Autodesk Inventor part; units mm, degrees
ref_plane "Work Plane1" through (0, 3.95, 0) normal (0, 1, 0) x (1, 0, 0)
ref_plane "Work Plane2" through (0, 4.1, 0) normal (0, 1, 0) x (1, 0, 0)
ref_plane "YZ Plane" through (0, 0, 0) normal (1, 0, 0) x (0, 1, 0)
sketch "Sketch1" plane through (0, 0, 0) normal (0, 1, 0) x (-1, 0, 0)
  circle A0 centre (0, 0) radius 2.5
  circle A1 centre (0, 0) radius 3.65
  dimension "d0" = 5
  dimension "d1" = 7.3
extrude "Extrusion1" add sketch "Sketch1" along normal blind 5.2
ref_plane "Work Plane1" through (0, 3.95, 0) normal (0, 1, 0) x (1, 0, 0)
sketch "Sketch2" plane through (0, 3.95, 0) normal (0, 1, 0) x (1, 0, 0)
  circle A0 centre (0, 0) radius 2.5
  circle A1 centre (0, 0) radius 1.2
  dimension "d5" = 2.4
extrude "Extrusion2" add sketch "Sketch2" against normal blind 1
ref_plane "Work Plane2" through (0, 4.1, 0) normal (0, 1, 0) x (1, 0, 0)
sketch "Sketch3" plane through (0, 4.1, 0) normal (0, 1, 0) x (1, 0, 0)
  line L0 (5.5656, 0) -> (-5.5656, 0) construction
  circle A0 centre (0, 16.05) radius 2
  line L1 (1.9896, 16.2533) -> (3.65, 0)
  circle A1 centre (0, 0) radius 3.65
  line L2 (-1.9896, 16.2533) -> (-3.65, 0)
  line L3 (0, 16.05) -> (0, 18.05)
  line L4 (0, 3.65) -> (0, -3.65) construction
  circle A2 centre (0, -16.05) radius 2
  line L5 (1.9896, -16.2533) -> (3.65, 0)
  line L6 (-1.9896, -16.2533) -> (-3.65, 0)
  line L7 (0, -16.05) -> (0, -18.05)
  point P0 (0, 0)
  point P1 (-3.5746, -0.738)
  point P2 (3.5746, -0.738)
  point P3 (-3.5746, 0.738)
  point P4 (3.5746, 0.738)
  dimension "d9" = 18.05
  dimension "d10" = 4
extrude "Extrusion3" add sketch "Sketch3" against normal blind 2.3 contours A0 | A0 L1 A1 L2 | L5 A2 L6 A1 | A2
sketch "Sketch4" plane through (0, 4.1, 0) normal (0, 1, 0) x (1, 0, 0)
  circle A0 centre (0, -15.6) radius 0.5
  point P0 (0, 0)
  dimension "d13" = 1
  dimension "d14" = 15.6
extrude "Extrusion4" cut sketch "Sketch4" against normal through all
properties part number "Servo_small_top"
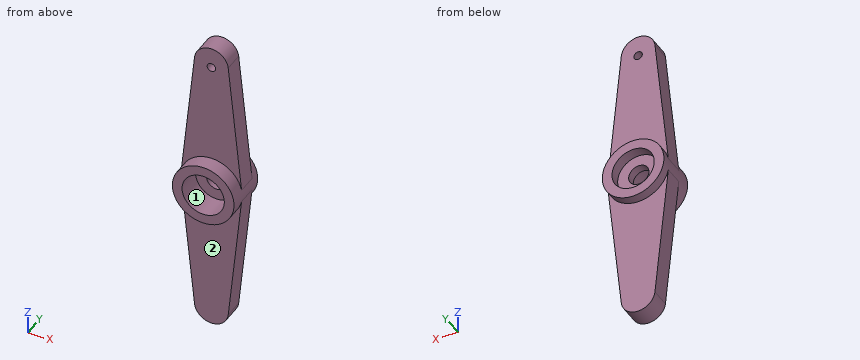
CAD build for the part. Positions are in the model's coordinates, mm. Face numbers are marked on the shaded views. Give positions to 0.01 mm unless a question says otherwise; leave off trailing zeros. Order: outer loops, then holes, each group sorted by start corner. A loop starts at its lowest first (then second) coordinate and runs counter-clockwise, first axis right, second up. Notation, with made-up numbers: (-4, 84.5) - (55, 84.5) arc R21 cw to (55, 117.5) - close; hole circle Ø11 at (72.25, 74). An arc over 180 degrees is marked (long way). Write each question's results on one line, items separated by ' | '.
1. Saw through at B-B on x = 0. List the corners of the cut face in (y, z).
Calculated:
outline: (0, -3.65) - (1.8, -3.65) - (1.8, -18.05) - (4.1, -18.05) - (4.1, -3.65) - (5.2, -3.65) - (5.2, -2.5) - (3.95, -2.5) - (3.95, -1.2) - (2.95, -1.2) - (2.95, -2.5) - (0, -2.5) - close; (0, 2.5) - (2.95, 2.5) - (2.95, 1.2) - (3.95, 1.2) - (3.95, 2.5) - (5.2, 2.5) - (5.2, 3.65) - (4.1, 3.65) - (4.1, 15.1) - (1.8, 15.1) - (1.8, 3.65) - (0, 3.65) - close; (1.8, 16.1) - (4.1, 16.1) - (4.1, 18.05) - (1.8, 18.05) - close
2. Pin check, flat tips, straight feed: pin 1 (2 mm diameter, centred on x = -1.5, z = 13.5, fed in from -Y); pin 2 (3 mm diameter, centred on x = 0, z = 0, fed in from +Y); pin 3 (1 mm diameter, centred on y = 3.5, z = 4, fed in from -X). Stop position of each tip, or through.
Calculated:
pin 1: stops at y = 1.8 | pin 2: stops at y = 3.95 | pin 3: stops at x = -3.29
3. Saw through at A-A on z = 0. List the corners of the cut face in (x, y).
Calculated:
outline: (-3.65, 0) - (-2.5, 0) - (-2.5, 2.95) - (-1.2, 2.95) - (-1.2, 3.95) - (-2.5, 3.95) - (-2.5, 5.2) - (-3.65, 5.2) - close; (1.2, 2.95) - (2.5, 2.95) - (2.5, 0) - (3.65, 0) - (3.65, 5.2) - (2.5, 5.2) - (2.5, 3.95) - (1.2, 3.95) - close
4. Saw through at D-D on z = 15.6. List the corners of the cut face in (x, y).
Calculated:
outline: (-2.06, 1.8) - (-0.5, 1.8) - (-0.5, 4.1) - (-2.06, 4.1) - close; (0.5, 1.8) - (2.06, 1.8) - (2.06, 4.1) - (0.5, 4.1) - close
5. Probe L1, parallel to Z at x = 0, y = 3.45; L2, parallel to Z at x = 0, y = 2.45; L3, parallel to Z at x = 0, y = 4.8. List the from-to ranges inside material, lowest first. Write a range as from..to.
Calculated:
L1: z = -18.05..-1.2, 1.2..15.1, 16.1..18.05 | L2: z = -18.05..-2.5, 2.5..15.1, 16.1..18.05 | L3: z = -3.65..-2.5, 2.5..3.65
6. Pull direction Z, two halves, no side cores. Call the marked faces 1 and 2: released by +Z, released by -Z, zero draft, split by the parting line, or undercut.
Calculated:
face 1: undercut | face 2: zero draft
7. Saw through at C-C on y = 0.95. List the corners of the cut face in (x, z), and give its area (3 significant figures).
Calculated:
outline: circle Ø7.3 at (0, 0); hole circle Ø5 at (0, 0) | area: 22.2 mm2
